```python
from build123d import *

# Parameters (mm, degrees)
SKETCH_1_R               = 47.25
SKETCH_1_R_2             = 38
SKETCH_1_R_3             = 3.1
EXTRUDE_1_DEPTH          = 3
CUT_EXTRUDE_1_DEPTH      = 67.888900425
CUT_EXTRUDE_1_DEPTH_BACK = 67.888900425
EXTRUDE_2_DEPTH          = 3
FILLET_1_R               = 1
CUT_EXTRUDE_2_DEPTH      = 82.883401917
CUT_EXTRUDE_2_DEPTH_BACK = 82.883401917
FILLET_2_R               = 0.5
CHAMFER_1_SIZE           = 0.5
CUT_EXTRUDE_3_DEPTH      = 82.883401775
CUT_EXTRUDE_3_DEPTH_BACK = 82.883401775
SKETCH_7_R               = 1.5
CUT_EXTRUDE_4_DEPTH      = 82.883401775
CUT_EXTRUDE_4_DEPTH_BACK = 82.883401775
SKETCH_8_R               = 1.5


with BuildPart() as part:
    # 草图1 → 凸台-拉伸1 (new body)
    with BuildSketch(Plane(origin=(0, 0, 0), x_dir=(1, 0, 0), z_dir=(0, 1, 0))):
        with Locations(Location((0, 0, 0), (0, 0, 270))):
            Circle(SKETCH_1_R)
        with Locations(Location((0, 0, 0), (0, 0, 270))):
            Circle(SKETCH_1_R_2, mode=Mode.SUBTRACT)
        with Locations(Location((-16.264045876, 39.264880132, 0), (0, 0, 270))):
            Circle(SKETCH_1_R_3, mode=Mode.SUBTRACT)
        with Locations(Location((16.264045876, 39.264880132, 0), (0, 0, 270))):
            Circle(SKETCH_1_R_3, mode=Mode.SUBTRACT)
        with Locations(Location((39.264880132, 16.264045876, 0), (0, 0, 270))):
            Circle(SKETCH_1_R_3, mode=Mode.SUBTRACT)
        with Locations(Location((39.264880132, -16.264045876, 0), (0, 0, 270))):
            Circle(SKETCH_1_R_3, mode=Mode.SUBTRACT)
        with Locations(Location((16.264045876, -39.264880132, 0), (0, 0, 270))):
            Circle(SKETCH_1_R_3, mode=Mode.SUBTRACT)
        with Locations(Location((-16.264045876, -39.264880132, 0), (0, 0, 270))):
            Circle(SKETCH_1_R_3, mode=Mode.SUBTRACT)
        with Locations(Location((-39.264880132, -16.264045876, 0), (0, 0, 270))):
            Circle(SKETCH_1_R_3, mode=Mode.SUBTRACT)
        with Locations(Location((-39.264880132, 16.264045876, 0), (0, 0, 270))):
            Circle(SKETCH_1_R_3, mode=Mode.SUBTRACT)
    extrude(amount=EXTRUDE_1_DEPTH)

    # 草图4 → 切除-拉伸1 (cut, two sides: drawn at the far end of the back side and taken through both)
    with BuildSketch(Plane(origin=(0, 3, 0), x_dir=(1, 0, 0), z_dir=(0, 1, 0)).offset(-CUT_EXTRUDE_1_DEPTH_BACK)):
        with BuildLine():
            Line((43.840620434, 12.727922061), (44.719682329, 13.606983957))
            ThreePointArc((44.719682329, 13.606983957), (45.806880456, 15.618172507), (45.614922333, 17.896336511))
            Line((45.614922333, 17.896336511), (84.379499133, 11.829199362))
            Line((84.379499133, 11.829199362), (6.001901693, -69.182953765))
            Line((6.001901693, -69.182953765), (-17.896336511, -45.614922333))
            ThreePointArc((-17.896336511, -45.614922333), (-15.618172507, -45.806880456), (-13.606983957, -44.719682329))
            Line((-13.606983957, -44.719682329), (-12.727922061, -43.840620434))
            ThreePointArc((-12.727922061, -43.840620434), (-9.899494937, -42.669047558), (-7.071067812, -43.840620434))
            Line((-7.071067812, -43.840620434), (6.363961031, -57.275649276))
            ThreePointArc((6.363961031, -57.275649276), (7.778174593, -57.861435714), (9.192388155, -57.275649276))
            Line((9.192388155, -57.275649276), (57.275649276, -9.192388155))
            ThreePointArc((57.275649276, -9.192388155), (57.861435714, -7.778174593), (57.275649276, -6.363961031))
            Line((57.275649276, -6.363961031), (43.840620434, 7.071067812))
            ThreePointArc((43.840620434, 7.071067812), (42.669047558, 9.899494937), (43.840620434, 12.727922061))
        make_face()
    extrude(amount=CUT_EXTRUDE_1_DEPTH + CUT_EXTRUDE_1_DEPTH_BACK, mode=Mode.SUBTRACT)

    # 草图5 → 凸台-拉伸2 (add)
    with BuildSketch(Plane.XZ):
        with BuildLine():
            Line((57.275649276, 6.363961031), (43.840620434, -7.071067812))
            ThreePointArc((43.840620434, -7.071067812), (33.021886933, 33.021886933), (-7.071067812, 43.840620434))
            Line((-7.071067812, 43.840620434), (6.363961031, 57.275649276))
            ThreePointArc((6.363961031, 57.275649276), (7.778174593, 57.861435714), (9.192388155, 57.275649276))
            Line((9.192388155, 57.275649276), (57.275649276, 9.192388155))
            ThreePointArc((57.275649276, 9.192388155), (57.861435714, 7.778174593), (57.275649276, 6.363961031))
        make_face()
    extrude(amount=-EXTRUDE_2_DEPTH)

    # 圆角1
    fillet_1_edges = [part.edges().sort_by_distance(p)[0] for p in [
        (45.109607697, 1.5, -14.060078003),
        (-14.060078003, 1.5, 45.109607697),
    ]]
    fillet(fillet_1_edges, radius=FILLET_1_R)

    # 草图6 → 切除-拉伸2 (cut, two sides: drawn at the far end of the back side and taken through both)
    with BuildSketch(Plane.XZ.offset(-CUT_EXTRUDE_2_DEPTH_BACK)):
        Polygon((29.839906166, 34.082546853), (34.082546853, 29.839906166), (35.355339059, 31.112698372), (31.112698372, 35.355339059), align=None)
    extrude(amount=CUT_EXTRUDE_2_DEPTH + CUT_EXTRUDE_2_DEPTH_BACK, mode=Mode.SUBTRACT)

    # 圆角2
    fillet_2_edges = [part.edges().sort_by_distance(p)[0] for p in [
        (34.082546853, 1.5, 29.839906166),
        (31.112698372, 1.5, 35.355339059),
        (35.355339059, 1.5, 31.112698372),
        (29.839906166, 1.5, 34.082546853),
    ]]
    fillet(fillet_2_edges, radius=FILLET_2_R)

    # 倒角1
    chamfer_1_edges = [part.edges().sort_by_distance(p)[0] for p in [
        (57.861435714, 0, 7.778174593),
        (7.778174593, 0, 57.861435714),
        (7.778174593, 3, 57.861435714),
        (57.861435714, 3, 7.778174593),
        (-33.410795411, 3, -33.410795411),
        (-33.410795411, 0, -33.410795411),
        (44.267555216, 0, -13.154856844),
        (-14.055418364, 0, 44.959744811),
        (44.959744811, 0, -14.055418364),
        (44.267555216, 3, -13.154856844),
        (-14.055418364, 3, 44.959744811),
        (44.959744811, 3, -14.055418364),
        (34.718942956, 0, 30.476302269),
        (31.96122651, 0, 31.96122651),
        (30.476302269, 0, 34.718942956),
        (19.975766569, 0, 46.492270863),
        (30.905591591, 0, 35.355339059),
        (35.355339059, 0, 30.905591591),
        (34.718942956, 3, 30.476302269),
        (19.975766569, 3, 46.492270863),
        (30.476302269, 3, 34.718942956),
        (31.96122651, 3, 31.96122651),
        (30.905591591, 3, 35.355339059),
        (35.355339059, 3, 30.905591591),
        (34.082546853, 0, 30.047012947),
        (34.082546853, 3, 30.047012947),
        (30.047012947, 0, 34.082546853),
        (30.047012947, 3, 34.082546853),
        (-0.353553391, 3, 50.558134855),
        (46.492270863, 0, 19.975766569),
        (50.558134855, 3, -0.353553391),
        (-13.154856844, 0, 44.267555216),
        (-9.899494937, 0, 42.669047558),
        (-0.353553391, 0, 50.558134855),
        (46.492270863, 3, 19.975766569),
        (50.558134855, 0, -0.353553391),
        (42.669047558, 0, -9.899494937),
        (42.669047558, 3, -9.899494937),
        (-9.899494937, 3, 42.669047558),
        (-13.154856844, 3, 44.267555216),
    ]]
    chamfer(chamfer_1_edges, length=CHAMFER_1_SIZE - 0.0001)  # a hair under: the kernel refuses the full size

    # 草图7 → 切除-拉伸3 (cut, two sides: drawn at the far end of the back side and taken through both)
    with BuildSketch(Plane.XZ.offset(-CUT_EXTRUDE_3_DEPTH_BACK)):
        with Locations(Location((13.678623105, 47.053925479, 0), (0, 0, 270))):
            Circle(SKETCH_7_R)
    extrude(amount=CUT_EXTRUDE_3_DEPTH + CUT_EXTRUDE_3_DEPTH_BACK, mode=Mode.SUBTRACT)

    # 草图8 → 切除-拉伸4 (cut, two sides: drawn at the far end of the back side and taken through both)
    with BuildSketch(Plane.XZ.offset(-CUT_EXTRUDE_4_DEPTH_BACK)):
        with Locations(Location((47.053925479, 13.678623105, 0), (0, 0, 270))):
            Circle(SKETCH_8_R)
    extrude(amount=CUT_EXTRUDE_4_DEPTH + CUT_EXTRUDE_4_DEPTH_BACK, mode=Mode.SUBTRACT)


solid = part.part
```
The listing builds one solid part. Answer for the finished solid, in the listing's coordinates (mm). A direction names the side the tool comes from. Round coordinates to 2 decimals unless told otherwise and drop trailing zeros. Write each loop counter-clockwise with the first axis right and the second up, starting at its lowest first coordinate (ties: lowest second). Pieces come first, ordered by that corner, then holes. Notation, with made-up numbers: (12, -4) -> (46, -4) arc R6 ccw to (46, 0) -> close; hole circle Ø7 at (-30, 60). An arc over 180 degrees is marked (long way). Answer as a JSON object with one key per item and string values. Group by question number.
Q1. Section A-A (x = 0) is taken. Write down the section's boundary in (y, z).
Q2. Determine the mould class of faces 1 (the face through (-32.197, 0.142, -34.092)), 2 (the face through (31.76, 0.25, 31.81)), 3 (the face through (-0.268, 2.754, 50.285)) for opening direction Z: pulls with the +Z half, pulls with the -Z half, needs draft (parallel to the pull), parting line crosses it, or undercut.
Q3. Straight lines are drawn through the part: line 1 along X through (y, z) = (0.7, -14.5); line 2 along Z through (x, y) = (-18.5, 1.7); line 3 along Z through (x, y) = (-40.5, 2.85). For each, find the intervals that lie inside material, in ascending order.
Q4. Each of these flat-tipped pins is pushed along its axis until it touches: pin 1 Ø8 at (x, z) = (39.26, -16.26) entering from -Y; pin 2 Ø1.5 at (y, z) = (1.5, -11.5) entering from -X; pin 3 Ø5 at (x, z) = (39.26, 16.26) entering from +Y; pin 4 Ø1 at (y, z) = (2.5, 26.5) entering from -X. Where does it stop, or does it pass through?
Q5. Section C-C (y = 1.35) is taken. Count the separate pieces of the cut face and the enclosed holes in it, plus the area to 3 significant figures.
Q6. Section B-B (z = 0) is taken. Write down the section's boundary in (x, y), plus the area to 3 significant figures.
Q7. Which of the six approach directions +Z, -Z, +X, -X, +Y, -Y give full straight-line access (tool end or side, diameter ignored) to faces 4 (the face through (36.515, 1.479, 17.695)), 5 (the face through (31.76, 2.75, 31.81))?
Check values:
{
 "1": {"outline": "(0, -46.75) -> (0.5, -47.25) -> (2.5, -47.25) -> (3, -46.75) -> (3, -38) -> (0, -38) -> close; (0, 38) -> (3, 38) -> (3, 50.2) -> (2.5, 50.91) -> (0.5, 50.91) -> (0, 50.2) -> close"},
 "2": {"face 1": "parting line crosses it", "face 2": "undercut", "face 3": "pulls with the +Z half"},
 "3": {"line 1": "-44.97 to -41.81, -36.72 to -35.12, 35.12 to 36.72, 41.81 to 44.96", "line 2": "-43.48 to -41.41, -37.12 to -33.19, 33.19 to 37.12, 41.41 to 43.48", "line 3": "-23.65 to -19.11, -13.42 to 13.42, 19.11 to 23.65"},
 "4": {"pin 1": "y = 0", "pin 2": "x = -46.01", "pin 3": "through", "pin 4": "x = -39.45"},
 "5": {"separate pieces": "1", "enclosed holes": "11", "area": "2,510 mm^2"},
 "6": {"outline": "(-47.25, 0.5) -> (-46.75, 0) -> (-38, 0) -> (-38, 3) -> (-46.75, 3) -> (-47.25, 2.5) -> close; (38, 0) -> (50.2, 0) -> (50.91, 0.5) -> (50.91, 2.5) -> (50.2, 3) -> (38, 3) -> close", "area": "65.9 mm^2"},
 "7": {"face 4": "+Y, -Y", "face 5": "+Y"}
}
